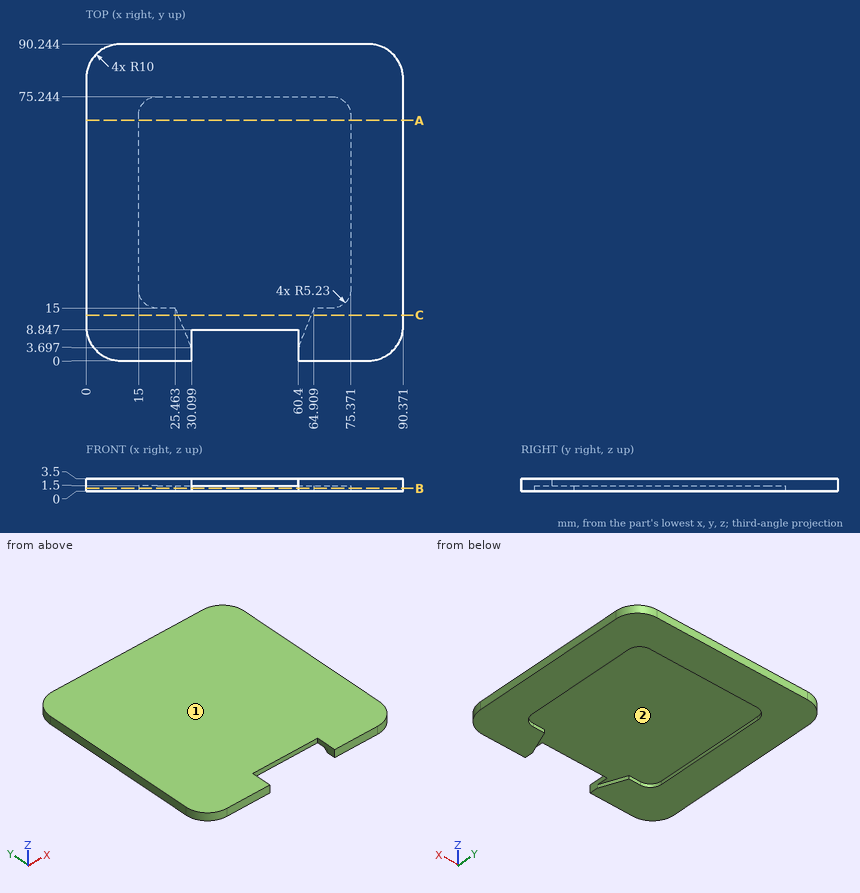
Geometry: see drawing. Coordinates: mm, zero at the bounding-box minimum. Coordinates: 2 decimals unless noted, no trailing zeros. Loops run counter-clockwise (first coordinate to the right, second up) from the corner with the lowest first, then second, coordinate; pieces in that order, holes last. Notation, with made-up numbers: M -11,-35 L -7,-35 A23 cw -7,0 Z; hole C 16.25,46.5 d1. An arc over 180 degrees is marked long. Answer in a Markdown table with one row per item.
1. Draft query along Y for the marked faces 1 and 2. Return one class per face: pulls with the +Y half, pulls with the -Y half, needs draft (parallel to the pull), parting line crosses it, or undercut.
Response:
| item | result |
|---|---|
| face 1 | needs draft |
| face 2 | undercut |
2. Section C-C, the plane y = 13. Output: boundary loops of the cut face in (x, z).
Response:
| item | result |
|---|---|
| outline | M 0,0 L 26.28,0 L 26.28,1.5 L 64.11,1.5 L 64.11,0 L 90.37,0 L 90.37,3.5 L 0,3.5 Z |
3. Material intervals for line 1 (X direction, y = 29, z = 1); line 2 (Y direction, x = 36.5, z = 2.05); line 3 (Z direction, x = 26, y = 26), sorted ascending.
Response:
| item | result |
|---|---|
| line 1 | x = 0 to 15, 75.37 to 90.37 |
| line 2 | y = 8.85 to 90.24 |
| line 3 | z = 1.5 to 3.5 |
4. Section A-A, the plane y = 68.5. Output: boundary loops of the cut face in (x, z), then the cut area to 3 significant figures.
Response:
| item | result |
|---|---|
| outline | M 0,0 L 15,0 L 15,1.5 L 75.37,1.5 L 75.37,0 L 90.37,0 L 90.37,3.5 L 0,3.5 Z |
| area | 226 mm2 |
5. Section B-B, the plane z = 0.8. Output: boundary loops of the cut face in (x, y).
Response:
| item | result |
|---|---|
| outline | M 0,10 A10 ccw 10,0 L 30.1,0 L 30.1,3.7 L 25.46,15 L 20.23,15 A5.23 cw 15,20.23 L 15,70.01 A5.23 cw 20.23,75.24 L 70.14,75.24 A5.23 cw 75.37,70.01 L 75.37,20.23 A5.23 cw 70.14,15 L 64.91,15 L 60.4,3.7 L 60.4,0 L 80.37,0 A10 ccw 90.37,10 L 90.37,80.24 A10 ccw 80.37,90.24 L 10,90.24 A10 ccw 0,80.24 Z |
6. First-contact query: pin 1 (10 mm diameter, centred on x = 63, y = 24, fed in from -Z); pin 2 (1 mm diameter, centred on x = 39, z = 2, fed in from -Y); pin 3 (1 mm diameter, centred on y = 2.5, z = 2, fed in from +X). Flat tips, straight axial feed; report the tip coordinate or a pass-through.
Response:
| item | result |
|---|---|
| pin 1 | stops at z = 1.5 |
| pin 2 | stops at y = 8.85 |
| pin 3 | stops at x = 87.51 |
